Answer from the drawing. Dimensions are ordinates in mm from the lowest x, y and z of the part. A direction names the side the tool comes from. Coordinates: 2 decimals unless noted, no trailing zeros. Write each loop counter-clockwise with the first axis right and the second up, starting at its lowest first coordinate (ties: lowest second). Pieces come first, ordered by that corner, then holes. Notation, with made-up numbers: (-39, 64.5) -> (2, 64.5) arc R31 ccw to (2, 93.5) -> close; hole circle Ø6 at (5, 70). An arc over 180 degrees is marked (long way). One line per item, written item: value. Start each with the question number.
1. For a pull along X with two mould halves and no side action, classify the marked faces 1, 2 and 3 as pulls with the +X half, pulls with the -X half, needs draft (parallel to the pull), parting line crosses it, or undercut.
2. Given P1, Ø5, axis at x = 6.5, z = 8, coming from the +Y side; P2, Ø5, axis at x = 3, y = 9.5, coming from the -Z side; P3, Ø1.5, axis at x = 2.52, y = 11.5, coming from the -Z side; P4, Ø4, axis at y = 11.5, z = 7.5, coming from the -X side, each flat-ended and moving along its own axis, determine where each tip first touches the part or whether it passes through.
3. Consider line 1 along Z through (x, y) = (2.5, 1.25); line 2 along X through (y, z) = (1.05, 7.5); line 3 along Y through (x, z) = (0.5, 14.75). Determine where each line is inside the solid, lowest interval first.
4. Find section A-A, the plane z = 14. Write down the section's boundary in (x, y) (1 decimal).
5. Find section D-D, the plane z = 7.5. State how many separate pieces and enclosed holes the cut face has.
6. Find section B-B, the plane y = 11.5. Write down the section's boundary in (x, z).
7. For the marked faces 4 and 5, determine the directions among +Z, -Z, +X, -X, +Y, -Y from which every point of the face is accessible in a straight line to the end or side of a thin tool.
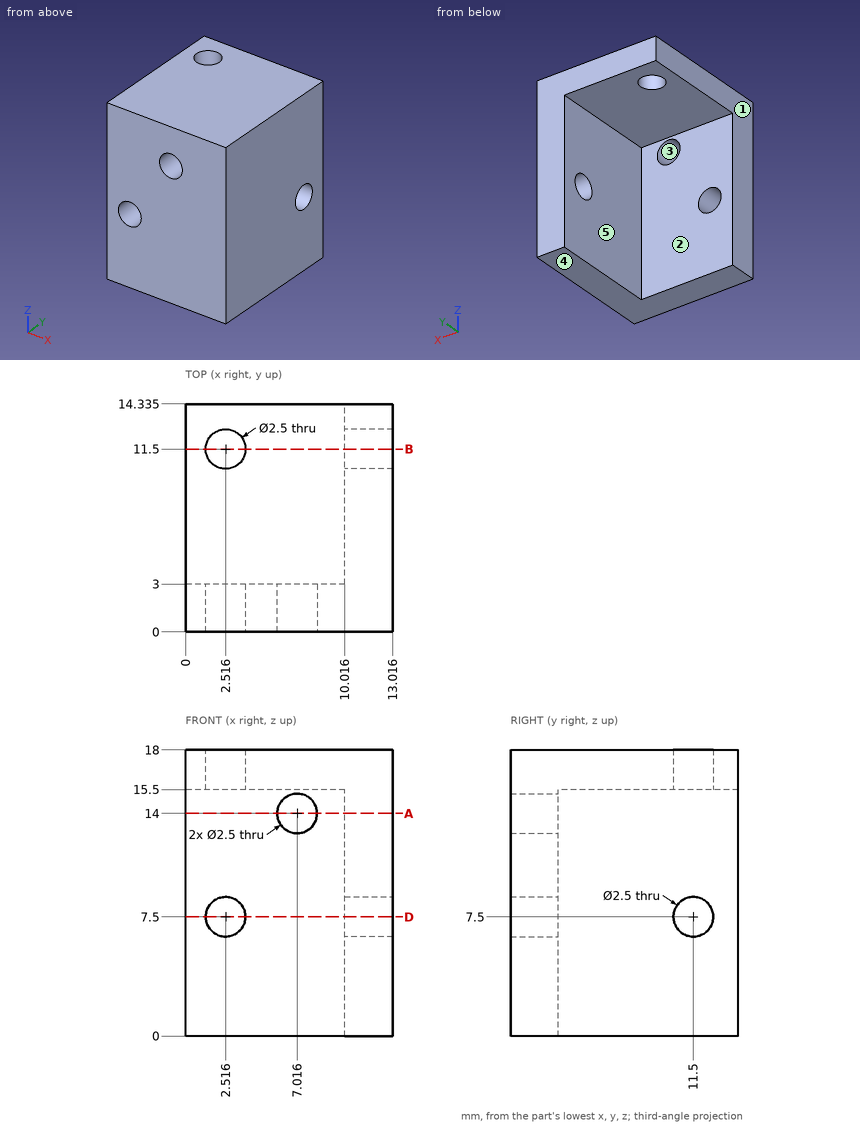
Answer block:
1. face 1: pulls with the -X half
1. face 2: needs draft
1. face 3: undercut
2. P1: stops at y = 3
2. P2: stops at z = 15.5
2. P3: passes through
2. P4: stops at x = 10.02
3. line 1: z = 0 to 6.25, 8.75 to 18
3. line 2: x = 0 to 1.27, 3.77 to 13.02
3. line 3: y = 0 to 3
4. outline: (0, 0) -> (5.8, 0) -> (5.8, 3) -> (0, 3) -> close; (8.3, 0) -> (13, 0) -> (13, 14.3) -> (10, 14.3) -> (10, 3) -> (8.3, 3) -> close
5. separate pieces: 3
5. enclosed holes: 0
6. outline: (0, 15.5) -> (1.27, 15.5) -> (1.27, 18) -> (0, 18) -> close; (3.77, 15.5) -> (10.02, 15.5) -> (10.02, 8.75) -> (13.02, 8.75) -> (13.02, 18) -> (3.77, 18) -> close; (10.02, 0) -> (13.02, 0) -> (13.02, 6.25) -> (10.02, 6.25) -> close
7. face 4: -Z, +X, -X, +Y, -Y
7. face 5: -Z, -X, +Y
